Geometry check sheet. Reference: drawing and pictorial views, mm from the part's lowest x, y, z. A direction names the side the tool comes from. Coordinates: 2 decimals unless noted, no trailing zeros. Write each loop counter-clockwise with the first axis right and the second up, starting at its lowest first coordinate (ties: lowest second). Pieces come first, ordered by that corner, then holes. Notation, with made-up numbers: M 36.5,1 L 61.5,1 A30 ccw 61.5,40 Z; hole C 67,-18.5 d8. An arc over 180 degrees is marked long. One line per item, written item: value.
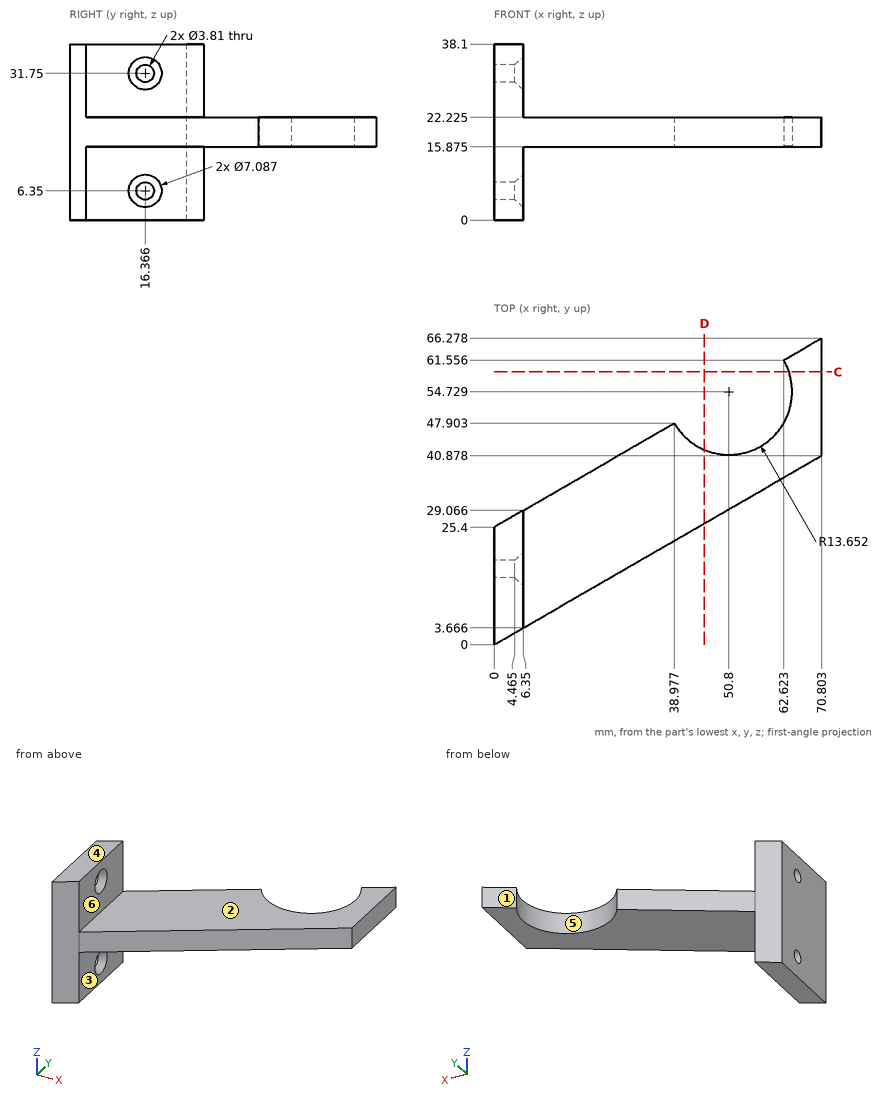
Item 1: Access from +Z, -Z, +X, -X, +Y, -Y to the whole of each face (thin tool, end or side, straight path). Record for the marked faces 1, 2 and 3.
The answers:
face 1: +Z, -Z, -X, +Y
face 2: +Z, +X, +Y, -Y
face 3: -Z, +X, +Y, -Y
Item 2: Cross-section at C-C, the plane y = 59. Enter the section's corners in (x, z) (1 decimal).
The answers:
outline: M 63.8,15.9 L 70.8,15.9 L 70.8,22.2 L 63.8,22.2 Z
Item 3: Cross-section at D-D, the plane x = 45.5. Enter the section's corners in (y, z) (1 decimal).
The answers:
outline: M 26.3,15.9 L 42.1,15.9 L 42.1,22.2 L 26.3,22.2 Z
Item 4: Draft check along X on the marked faces 4, 5 and 6. Enter one of: released by +X, released by -X, zero draft, split by the parting line, or undercut.
The answers:
face 4: zero draft
face 5: undercut
face 6: released by +X
Item 5: Go/stop test with flat-tipped pins: P1, Ø12.5, axis at y = 18.5, z = 6.5, coming from the +X side; P2, Ø12, axis at x = 60, y = 33.5, coming from the -Z side (1 decimal); P3, Ø10, axis at x = 54, z = 19, coming from the -Y side. Record where each tip stops, or that it passes through.
The answers:
P1: stops at x = 6.35
P2: stops at z = 15.9
P3: stops at y = 28.29
Item 6: Scan lines: line 1 (Z direction, x = 6, y = 15) (1 decimal); line 2 (Z direction, x = 36.5, y = 33) (1 decimal); line 3 (Y direction, x = 2.85, z = 6.35) (1 decimal). Record each from-to range of solid material in increasing order.
The answers:
line 1: z = 0 to 3.4, 9.3 to 28.8, 34.7 to 38.1
line 2: z = 15.9 to 22.2
line 3: y = 1.6 to 14.5, 18.3 to 27
